```python
from build123d import *

# Parameters (mm, degrees)
PAD001_DEPTH    = 1.4
SKETCH012_R     = 2.25
POCKET_DEPTH    = 5
SKETCH011_W     = 14
SKETCH011_H     = 14
POCKET005_DEPTH = 5


with BuildPart() as part:
    # Sketch002 → Pad001 (new body)
    with BuildSketch(Plane.XY):
        Polygon((0.5, 75.7), (48.125, 75.7), (48.125, 85.225), (67.175, 85.225), (67.175, 89.9875), (85.225, 89.9875), (85.225, 85.225), (104.275, 85.225), (104.275, 80.4625), (142.375, 80.4625), (142.375, 16.647033), (164.08137, 6.943809), (148.940768, -26.926121), (131.957481, -19.334219), (104.444214, -13.486094), (105.392449, -9.025), (86.225, -9.025), (86.225, -4.2625), (66.175, -4.2625), (66.175, -9.025), (48.125, -9.025), (48.125, 0.5), (0.5, 0.5), align=None)
        Polygon((111.504412, -12.916546), (125.198478, -15.827309), (128.109242, -2.133243), (114.415175, 0.777521), align=None, mode=Mode.SUBTRACT)
        Polygon((135.137374, -18.537583), (147.91848, -24.251018), (153.631915, -11.469912), (140.850809, -5.756478), align=None, mode=Mode.SUBTRACT)
        Polygon((142.911774, -1.146151), (155.69288, -6.859586), (161.406273, 5.921518), (148.625201, 11.634938), align=None, mode=Mode.SUBTRACT)
    extrude(amount=PAD001_DEPTH)

    # Sketch012 (on Face37 of Pad001) → Pocket (cut)
    with BuildSketch(Plane.XY.offset(1.4)):
        with Locations((28.575, 57.15)):
            Circle(SKETCH012_R)
        with Locations((28.575, 19.05)):
            Circle(SKETCH012_R)
        with Locations((104.775, 66.675)):
            Circle(SKETCH012_R)
        with Locations((104.775, 9.525)):
            Circle(SKETCH012_R)
    extrude(amount=-POCKET_DEPTH, mode=Mode.SUBTRACT)

    # Sketch011 (on Face37 of Pad001) → Pocket005 (cut)
    with BuildSketch(Plane.XY.offset(1.4)):
        with Locations((14.2875, 9.525)):
            Rectangle(SKETCH011_W, SKETCH011_H)
        with Locations((14.2875, 28.575)):
            Rectangle(SKETCH011_W, SKETCH011_H)
        with Locations((14.2875, 47.625)):
            Rectangle(SKETCH011_W, SKETCH011_H)
        with Locations((14.2875, 66.675)):
            Rectangle(SKETCH011_W, SKETCH011_H)
        with Locations((38.1, 9.525)):
            Rectangle(SKETCH011_W, SKETCH011_H)
        with Locations((38.1, 28.575)):
            Rectangle(SKETCH011_W, SKETCH011_H)
        with Locations((38.1, 47.625)):
            Rectangle(SKETCH011_W, SKETCH011_H)
        with Locations((38.1, 66.675)):
            Rectangle(SKETCH011_W, SKETCH011_H)
        with Locations((57.15, 0)):
            Rectangle(SKETCH011_W, SKETCH011_H)
        with Locations((57.15, 19.05)):
            Rectangle(SKETCH011_W, SKETCH011_H)
        with Locations((57.15, 38.1)):
            Rectangle(SKETCH011_W, SKETCH011_H)
        with Locations((57.15, 57.15)):
            Rectangle(SKETCH011_W, SKETCH011_H)
        with Locations((57.15, 76.2)):
            Rectangle(SKETCH011_W, SKETCH011_H)
        with Locations((76.2, 4.7625)):
            Rectangle(SKETCH011_W, SKETCH011_H)
        with Locations((76.2, 23.8125)):
            Rectangle(SKETCH011_W, SKETCH011_H)
        with Locations((76.2, 42.8625)):
            Rectangle(SKETCH011_W, SKETCH011_H)
        with Locations((76.2, 61.9125)):
            Rectangle(SKETCH011_W, SKETCH011_H)
        with Locations((76.2, 80.9625)):
            Rectangle(SKETCH011_W, SKETCH011_H)
        with Locations((95.25, 0)):
            Rectangle(SKETCH011_W, SKETCH011_H)
        with Locations((95.25, 19.05)):
            Rectangle(SKETCH011_W, SKETCH011_H)
        with Locations((95.25, 38.1)):
            Rectangle(SKETCH011_W, SKETCH011_H)
        with Locations((95.25, 57.15)):
            Rectangle(SKETCH011_W, SKETCH011_H)
        with Locations((95.25, 76.2)):
            Rectangle(SKETCH011_W, SKETCH011_H)
        with Locations((114.3, 14.2875)):
            Rectangle(SKETCH011_W, SKETCH011_H)
        with Locations((114.3, 33.3375)):
            Rectangle(SKETCH011_W, SKETCH011_H)
        with Locations((114.3, 52.3875)):
            Rectangle(SKETCH011_W, SKETCH011_H)
        with Locations((114.3, 71.4375)):
            Rectangle(SKETCH011_W, SKETCH011_H)
        with Locations((133.35, 19.05)):
            Rectangle(SKETCH011_W, SKETCH011_H)
        with Locations((133.35, 47.625)):
            Rectangle(SKETCH011_W, SKETCH011_H)
        with Locations((133.35, 71.4375)):
            Rectangle(SKETCH011_W, SKETCH011_H)
    extrude(amount=-POCKET005_DEPTH, mode=Mode.SUBTRACT)


with BuildPart() as part_1:
    # Body001 placement: moved
    add(part.part.moved(Location((0, 0, 5))))


solid = part_1.part
```
Can you work these out from the model? Positions are in its coordinate system, mm. A direction names the side the tool comes from. Give positions to 0.01 mm unless a question says otherwise; leave off trailing zeros. Loops run counter-clockwise (first coordinate to the right, second up) from the corner with the lowest first, then second, coordinate; pieces in that order, holes last. Notation, with made-up numbers: M -7.75,49.5 L 35.25,49.5 A18 ccw 35.25,74.5 Z; hole C -35,31.25 d3. An arc over 180 degrees is marked long. Use one line per item in the form item = value. Start each with the question number.
(1) I'm going to push flat-ended pins straight in: P1, Ø0.7, axis at x = 74.5, z = 6, coming from the -Y side; P2, Ø0.7, axis at x = 41.5, z = 5.5, coming from the -Y side; P3, Ø0.7, axis at x = 55.5, z = 5.5, coming from the +Y side (3 decimals). Where does each tip first touch, or does it pass through?
(2) On a 3-axis mill with a long thin cutter (end or side, diameter ignored), from which of +Z, -Z, +X, -X, +Y, -Y can I reach the whole of each face in a straight line? I mean faces 1 (the flat face through (150.735, -17.95, 5.69)), 2 (the flat face through (153.08, 11.86, 5.69)). Say none if no direction works.
(3) I want a section at D-D, the plane z = 5.5. State how many separate pieces and enclosed holes the cut face has, and give its area (3 significant figures).
(4) I want a section at B-B, the plane y = 57.15. Write out the boundary of the cut face in (x, z) (3 decimals), and give its area (3 significant figures).
(5) Thinking about a two-plate mould opening in Y: for faces 3 (the flat face through (118.39, -16.45, 5.69)), 4 (the flat face through (65, 32, 5)), 5 (the flat face through (149.21, -3.96, 5.69)), 6 (the cylindrical face through (102.527, 9.624, 5.71)), which applies, released by +Y, released by -Y, zero draft, split by the parting line, or undercut?
(6) I want a section at C-C, the plane y = 19.05. Write out the boundary of the cut face in (x, z) (3 decimals), and give its area (3 significant figures).
(7) I want a section at A-A, the plane x = 71.5. Write out the boundary of the cut face in (y, z), and give its area (4 significant figures).
(8) Please list where these lines run through material, in increasing order: line 1 (Y direction, x = 96.5, z = 5.7) (3 decimals); line 2 (Y direction, x = 76.5, z = 5.45); line 3 (Y direction, x = 43, z = 6.15) (3 decimals).
Worked out:
q1.P1 = -4.26
q1.P2 = 0.5
q1.P3 = 85.225
q2.face_1 = +Z, -Z
q2.face_2 = +Z, -Z, +X, +Y
q3.separate_pieces = 1
q3.enclosed_holes = 37
q3.area = 6,650 mm²
q4.outline = M 0.5,5 L 26.325,5 L 26.325,6.4 L 0.5,6.4 Z; M 30.825,5 L 50.15,5 L 50.15,6.4 L 30.825,6.4 Z; M 64.15,5 L 69.2,5 L 69.2,6.4 L 64.15,6.4 Z; M 83.2,5 L 88.25,5 L 88.25,6.4 L 83.2,6.4 Z; M 102.25,5 L 107.3,5 L 107.3,6.4 L 102.25,6.4 Z; M 121.3,5 L 142.375,5 L 142.375,6.4 L 121.3,6.4 Z
q4.area = 114 mm²
q5.face_3 = released by -Y
q5.face_4 = zero draft
q5.face_5 = undercut
q5.face_6 = undercut
q6.outline = M 0.5,5 L 26.325,5 L 26.325,6.4 L 0.5,6.4 Z; M 30.825,5 L 50.15,5 L 50.15,6.4 L 30.825,6.4 Z; M 64.15,5 L 69.2,5 L 69.2,6.4 L 64.15,6.4 Z; M 83.2,5 L 88.25,5 L 88.25,6.4 L 83.2,6.4 Z; M 102.25,5 L 107.3,5 L 107.3,6.4 L 102.25,6.4 Z; M 121.3,5 L 126.35,5 L 126.35,6.4 L 121.3,6.4 Z; M 140.35,5 L 142.375,5 L 142.375,6.4 L 140.35,6.4 Z
q6.area = 94.3 mm²
q7.outline = M -4.26,5 L -2.24,5 L -2.24,6.4 L -4.26,6.4 Z; M 11.76,5 L 16.81,5 L 16.81,6.4 L 11.76,6.4 Z; M 30.81,5 L 35.86,5 L 35.86,6.4 L 30.81,6.4 Z; M 49.86,5 L 54.91,5 L 54.91,6.4 L 49.86,6.4 Z; M 68.91,5 L 73.96,5 L 73.96,6.4 L 68.91,6.4 Z; M 87.96,5 L 89.99,5 L 89.99,6.4 L 87.96,6.4 Z
q7.area = 33.95 mm²
q8.line_1 = -9.025 to -7, 7 to 12.05, 26.05 to 31.1, 45.1 to 50.15, 64.15 to 69.2, 83.2 to 85.225
q8.line_2 = -4.26 to -2.24, 11.76 to 16.81, 30.81 to 35.86, 49.86 to 54.91, 68.91 to 73.96, 87.96 to 89.99
q8.line_3 = 0.5 to 2.525, 16.525 to 21.575, 35.575 to 40.625, 54.625 to 59.675, 73.675 to 75.7
